Design review of the part built by this model. Coordinates are the model's own, in mm. Give positions to 0.01 mm unless a question says otherwise; leave off trailing zeros. Write each loop counter-clockwise with the first axis right and the second up, starting at its lowest first coordinate (ties: lowest second). Pieces come first, ordered by that corner, then holes. Notation, with made-up numbers: M 65,72.25 L 116,72.25 A15 ccw 116,79.25 Z; hole C 38,73.25 d7. An arc over 180 degrees is marked long. Answer in a Markdown table with one row per item.
```python
from build123d import *

# Parameters (mm, degrees)
EXTRUDE_1_DEPTH = 3


with BuildPart() as part:
    # 草图1 → 凸台-拉伸1 (new body)
    with BuildSketch(Plane(origin=(0, 0, 0), x_dir=(1, 0, 0), z_dir=(0, 1, 0))):
        with BuildLine():
            Line((-55, -220), (-55, -300))
            ThreePointArc((-55, -300), (-69.644660941, -335.355339059), (-105, -350))
            Line((-105, -350), (-200, -350))
            ThreePointArc((-200, -350), (-235.355339059, -335.355339059), (-250, -300))
            Line((-250, -300), (-250, 300))
            ThreePointArc((-250, 300), (-235.355339059, 335.355339059), (-200, 350))
            Line((-200, 350), (200, 350))
            ThreePointArc((200, 350), (235.355339059, 335.355339059), (250, 300))
            Line((250, 300), (250, -300))
            ThreePointArc((250, -300), (235.355339059, -335.355339059), (200, -350))
            Line((200, -350), (105, -350))
            ThreePointArc((105, -350), (69.644660941, -335.355339059), (55, -300))
            Line((55, -300), (55, -220))
            ThreePointArc((55, -220), (0, -165), (-55, -220))
        make_face()
    extrude(amount=EXTRUDE_1_DEPTH)


solid = part.part
```
1) Add section C-C (x = 0). Write out the cut boundary in (y, z).
Geometry says:
| item | result |
|---|---|
| outline | M 0,-350 L 3,-350 L 3,165 L 0,165 Z |
2) The part is to be moulded in two halves that separate along X. For faces 1 (the face through (-69.258, 1.479, 334.964)), 2 (the face through (70.036, 1.479, 335.742)), 3 (the face through (-235.742, 1.479, -334.964)), 4 (the face through (235.742, 1.479, 334.964)), say which applies: released by +X, released by -X, zero draft, split by the parting line, or undercut.
Geometry says:
| item | result |
|---|---|
| face 1 | undercut |
| face 2 | undercut |
| face 3 | released by -X |
| face 4 | released by +X |
3) To check wall thickness, follow probe 1 along X at (y, z) = (1, 246.5); probe 2 along Z at (x, y) = (-3.5, 0.85); probe 3 along Z at (x, y) = (103.5, 0.25). State the ranges of each line that lie inside material, in increasing order. Write a range as [from, to].
Geometry says:
| item | result |
|---|---|
| probe 1 | [-250, -55], [55, 250] |
| probe 2 | [-350, 165.11] |
| probe 3 | [-350, 349.98] |
4) Add section A-A (y = 2.45). Write out the cut boundary in (x, z), and give its area (3 significant figures).
Geometry says:
| item | result |
|---|---|
| outline | M -250,-300 A50 ccw -200,-350 L 200,-350 A50 ccw 250,-300 L 250,300 A50 ccw 200,350 L 105,350 A50 ccw 55,300 L 55,220 A55 cw -55,220 L -55,300 A50 ccw -105,350 L -200,350 A50 ccw -250,300 Z |
| area | 328,000 mm^2 |
5) Add section B-B (z = 183). Write out the cut boundary in (x, y).
Geometry says:
| item | result |
|---|---|
| outline | M -250,0 L -40.69,0 L -40.69,3 L -250,3 Z; M 40.69,0 L 250,0 L 250,3 L 40.69,3 Z |
6) Insertion check: P1, Ø1.5, axis at x = 123.5, z = 195, coming from the -Y side. The pin has a flat end and moves straight along its axis. Give the tip position at first contact, or say it passes through.
Geometry says:
| item | result |
|---|---|
| P1 | y = 0 |
